from build123d import *

# Parameters (mm, degrees)
SKETCH_1_R          = 1.5
EXTRUDE_1_DEPTH     = 5
EXTRUDE_2_DEPTH     = 6
SKETCH_3_R          = 1.5
CUT_EXTRUDE_1_DEPTH = 5


with BuildPart() as part:
    # 草图1 → 凸台-拉伸1 (new body)
    with BuildSketch(Plane(origin=(0, 0, 0), x_dir=(1, 0, 0), z_dir=(0, 1, 0))):
        Circle(SKETCH_1_R)
    extrude(amount=EXTRUDE_1_DEPTH)

    # 草图2 → 凸台-拉伸2 (add)
    with BuildSketch(Plane(origin=(0, 5, 0), x_dir=(1, 0, 0), z_dir=(0, 1, 0))):
        Polygon((0, 2.309401077), (-2, 1.154700538), (-2, -1.154700538), (0, -2.309401077), (2, -1.154700538), (2, 1.154700538), align=None)
    extrude(amount=EXTRUDE_2_DEPTH)

    # 草图3 → 切除-拉伸1 (cut)
    with BuildSketch(Plane(origin=(0, 11, 0), x_dir=(1, 0, 0), z_dir=(0, 1, 0))):
        Circle(SKETCH_3_R)
    extrude(amount=-CUT_EXTRUDE_1_DEPTH, mode=Mode.SUBTRACT)


solid = part.part
Verification items for the finished model (mm, model axes). A direction names the side the tool comes from. Round coordinates to 2 decimals unless told otherwise and drop trailing zeros. Order: outer loops, then holes, each group sorted by start corner. A loop starts at its lowest first (then second) coordinate and runs counter-clockwise, first axis right, second up.
1. Release check for a two-part mould opening along X. For faces 4 (the cylindrical face through (-1.5, 8.54, -0.07)), 5 (the flat face through (0, 0, 0)), 6 (the flat face through (2, 8, 0)) record: +X half, -X half, draft (parallel to the pull), parting line (faces both ways), or undercut.
Final values:
face 4: undercut
face 5: draft
face 6: +X half
2. Access from +Z, -Z, +X, -X, +Y, -Y to the whole of each face (thin tool, end or side, straight path). Record for faces 1 (the flat face through (1.014, 7.958, -1.724)), 2 (the flat face through (0, 6, 0)), 3 (the flat face through (0, 5, 2)).
Final values:
face 1: -Z, +X, +Y, -Y
face 2: +Y
face 3: -Y
3. Thickness scan on L1, parallel to X at y = 8.3, z = 0; L2, parallel to Z at x = -0.4, y = 6.5; L3, parallel to Y at x = 1.25, z = -0.55. Record the ranges inside material, lowest first.
Final values:
L1: x = -2 to -1.5, 1.5 to 2
L2: z = -2.08 to -1.45, 1.45 to 2.08
L3: y = 0 to 6
4. Section check A-A on y = 9.75. Record the cut outline in (x, z).
Final values:
outline: (-2, -1.15) - (0, -2.31) - (2, -1.15) - (2, 1.15) - (0, 2.31) - (-2, 1.15) - close; hole circle Ø3 at (0, 0)
5. Go/stop test with a flat-tipped pin: P1, Ø1.8, axis at x = 0, z = 0, coming from the +Y side. Record where the tip stops, or that it passes through.
Final values:
P1: stops at y = 6
6. Section check B-B on z = 0. Record the cut outline in (x, y), then the cut area to 3 significant figures.
Final values:
outline: (-2, 5) - (-1.5, 5) - (-1.5, 0) - (1.5, 0) - (1.5, 5) - (2, 5) - (2, 11) - (1.5, 11) - (1.5, 6) - (-1.5, 6) - (-1.5, 11) - (-2, 11) - close
area: 24.0 mm2
7. Section check D-D on y = 1.25. Record the cut outline in (x, z), then the cut area to 3 significant figures.
Final values:
outline: circle Ø3 at (0, 0)
area: 7.07 mm2
8. Section check C-C on x = -0.65. Record the cut outline in (y, z), then the cut area to 3 significant figures.
Final values:
outline: (0, -1.35) - (5, -1.35) - (5, -1.93) - (11, -1.93) - (11, -1.35) - (6, -1.35) - (6, 1.35) - (11, 1.35) - (11, 1.93) - (5, 1.93) - (5, 1.35) - (0, 1.35) - close
area: 23.2 mm2
